from build123d import *

# Parameters (mm, degrees)
SKETCH3_R          = 2.352290117
CUT_EXTRUDE1_DEPTH = 10
CIRPATTERN1_COUNT  = 4
FILLET1_R          = 1


with BuildPart() as part:
    # Sketch2 → Revolve1 (revolve)
    with BuildSketch(Plane.XY):
        Polygon((0, 9.231240755), (0, -15.768759245), (10, -15.768759245), (14.214231209, -12.495683607), (14.214231209, -2.495683607), (6.923362893, -0.768759245), (1.2, -0.768759245), (1.2, 9.231240755), align=None)
    revolve(axis=Axis((0, 9.231240755, 0), (0, -1, 0)))

    # Sketch3 → Cut-Extrude1 (cut)
    with BuildSketch(Plane(origin=(0, 4.615620377, 0), x_dir=(1, 0, 0), z_dir=(0, 1, 0))):
        with Locations((0, -6.470406052)):
            Circle(SKETCH3_R)
    cut_extrude1 = extrude(amount=-CUT_EXTRUDE1_DEPTH, mode=Mode.SUBTRACT)

    # CirPattern1: Cut-Extrude1 ×4 about axis
    cirpattern1_axis = Axis((0, 0, 0), (0, 1, 0))
    for i in range(1, CIRPATTERN1_COUNT):
        add(cut_extrude1.rotate(cirpattern1_axis, i * 360 / CIRPATTERN1_COUNT), mode=Mode.SUBTRACT)

    # Fillet1
    fillet1_edges = [part.edges().sort_by_distance(p)[0] for p in [
        (-14.214231209, -2.495683607, 0),
        (-14.214231209, -12.495683607, 0),
    ]]
    fillet(fillet1_edges, radius=FILLET1_R)


solid = part.part
Design review of the part built by this model. Coordinates are the model's own, in mm. A direction names the side the tool comes from. Coordinates: 2 decimals unless noted, no trailing zeros. Write each loop counter-clockwise with the first axis right and the second up, starting at its lowest first coordinate (ties: lowest second). Pieces come first, ordered by that corner, then holes. Notation, with made-up numbers: (32, 62.5) - (52, 62.5) arc R12 ccw to (52, 70.5) - close; hole circle Ø5 at (6.5, 66). An arc over 180 degrees is marked (long way). One line per item, written item: value.
1) For faces 4 (the face through (0, 9.231, 0)), 5 (the face through (0.65, 4.3, 1.01)), list the 3-axis set-ups (+Z, -Z, +X, -X, +Y, -Y) from which the entire face can be reached by the end or side of a thin tool; tool diameter is ignored.
Answer sheet:
face 4: +Z, -Z, +X, -X, +Y
face 5: +Y
2) Add section A-A (y = 6.75). State the section outline as (x, z) points, plus the area to 3 significant figures.
Answer sheet:
outline: circle Ø2.4 at (0, 0)
area: 4.52 mm2
3) Insertion check: pin 1 (4 mm diameter, centred on x = -10, y = -2.5, fed in from +Z); pin 2 (2 mm diameter, centred on x = 3, y = -1.5, fed in from +Z); pin 3 (4 mm diameter, centred on x = 3, z = -2, fed in from +Y). Each pin has a flat end and moves straight along its axis. Give the tip position at first contact, or say it passes through.
Answer sheet:
pin 1: stops at z = 11.66
pin 2: stops at z = 13.52
pin 3: stops at y = -0.77
4) Mouldability with a two-part tool opening along X and no side actions: class faces 1 (the face through (6.56, -7.59, -12.61)), 2 (the face through (0, -15.769, 0)), 3 (the face through (4.14, -3.04, 0.31)) as +X half, -X half, draft (parallel to the pull), parting line (faces both ways), or undercut.
Answer sheet:
face 1: parting line
face 2: draft
face 3: undercut
5) To check wall thickness, follow probe 1 along X at (y, z) = (-3.35, 0); probe 2 along Z at (x, y) = (-0.25, -10.25). State the ranges of each line that lie inside material, in increasing order.
Answer sheet:
probe 1: x = -14.21 to -8.82, -4.12 to 4.12, 8.82 to 14.21
probe 2: z = -14.21 to 14.21
